```python
from build123d import *

# Parameters (mm, degrees)
SKETCH_1_W               = 20
SKETCH_1_H               = 149.015
SKETCH_1_R               = 2.15
EXTRUDE_1_DEPTH          = 10
SKETCH_2_W               = 20
SKETCH_2_H               = 20
EXTRUDE_2_DEPTH          = 40
SKETCH_3_W               = 20
SKETCH_3_H               = 20
EXTRUDE_3_DEPTH          = 18
CUT_EXTRUDE_1_DEPTH      = 10
CUT_EXTRUDE_1_DEPTH_BACK = 20
SKETCH_5_R               = 2.2
CUT_EXTRUDE_2_DEPTH      = 2
CUT_EXTRUDE_START        = -2
SKETCH_6_R               = 5
SKETCH_6_R_2             = 4.75
CUT_EXTRUDE_3_DEPTH      = 20
SKETCH_7_W               = 20
SKETCH_7_H               = 10
EXTRUDE_4_DEPTH          = 40
CUT_EXTRUDE_5_REACH      = 109.242


with BuildPart() as part:
    # 草图1 → 凸台-拉伸1 (new body)
    with BuildSketch(Plane.XY):
        with Locations((20.013762606, -57.295888527)):
            Rectangle(SKETCH_1_W, SKETCH_1_H)
        with Locations((20, -124.653388527)):
            Circle(SKETCH_1_R, mode=Mode.SUBTRACT)
    extrude(amount=EXTRUDE_1_DEPTH)

    # 草图2 → 凸台-拉伸2 (add)
    with BuildSketch(Plane.XY.offset(10)):
        with Locations((20.013762606, 7.211611473)):
            Rectangle(SKETCH_2_W, SKETCH_2_H)
    extrude(amount=EXTRUDE_2_DEPTH)

    # 草图3 → 凸台-拉伸3 (add)
    with BuildSketch(Plane(origin=(0, 0, 0), x_dir=(-1, 0, 0), z_dir=(0, 0, -1))):
        with Locations((-20.013762606, 7.211611473)):
            Rectangle(SKETCH_3_W, SKETCH_3_H)
    extrude(amount=EXTRUDE_3_DEPTH)

    # 草图4 → 切除-拉伸1 (cut, two sides: drawn at the far end of the back side and taken through both)
    with BuildSketch(Plane.XZ.offset(2.788388527).offset(-CUT_EXTRUDE_1_DEPTH_BACK)):
        Polygon((17.893762606, 50), (30.013762606, 50), (30.013762606, 10), align=None)
        Polygon((17.893762606, -18), (30.013762606, -18), (30.013762606, 0), align=None)
    extrude(amount=CUT_EXTRUDE_1_DEPTH + CUT_EXTRUDE_1_DEPTH_BACK, mode=Mode.SUBTRACT)

    # 草图5 → 切除-拉伸2 (cut)
    with BuildSketch(Plane.ZY.offset(-10.013762606)):
        with Locations(Location((14.7, 7.211611473, 0), (0, 0, 270))):
            Circle(SKETCH_5_R)
        with Locations(Location((40.7, 7.211611473, 0), (0, 0, 270))):
            Circle(SKETCH_5_R)
        with Locations(Location((-11.3, 7.211611473, 0), (0, 0, 270))):
            Circle(SKETCH_5_R)
    extrude(amount=-CUT_EXTRUDE_2_DEPTH, mode=Mode.SUBTRACT)

    # 草图6 → 切除-拉伸3 (cut)
    with BuildSketch(Plane.ZY.offset(-10.013762606).offset(CUT_EXTRUDE_START)):
        with Locations(Location((40.7, 7.211611473, 0), (0, 0, 270))):
            Circle(SKETCH_6_R)
        with Locations(Location((-11.3, 7.211611473, 0), (0, 0, 270))):
            Circle(SKETCH_6_R)
        with Locations(Location((14.7, 7.211611473, 0), (0, 0, 270))):
            Circle(SKETCH_6_R_2)
    extrude(amount=-CUT_EXTRUDE_3_DEPTH, mode=Mode.SUBTRACT)

    # 草图7 → 凸台-拉伸4 (add)
    with BuildSketch(Plane(origin=(0, 0, 0), x_dir=(-1, 0, 0), z_dir=(0, 0, -1))):
        with Locations((-20.013762606, -46.803388527)):
            Rectangle(SKETCH_7_W, SKETCH_7_H)
    extrude(amount=EXTRUDE_4_DEPTH)

    # 草图8 → 切除-拉伸5 (cut, up to next)
    with BuildSketch(Plane(origin=(0, -41.803388527, 0), x_dir=(1, 0, 0), z_dir=(0, 1, 0)), mode=Mode.PRIVATE) as cut_extrude_5_sk1:
        with BuildLine():
            Line((30.013762606, 20), (30.013762606, 40))
            Line((30.013762606, 40), (11.013762606, 40))
            ThreePointArc((11.013762606, 40), (19.239482102, 28.789433521), (30.013762606, 20))
        make_face()
    cut_extrude_5_tool1 = extrude(cut_extrude_5_sk1.sketch, amount=-CUT_EXTRUDE_5_REACH, mode=Mode.PRIVATE) & part.part
    add(cut_extrude_5_tool1.solids().sort_by_distance((23.14433, -41.803389, -32.776655))[0], mode=Mode.SUBTRACT)


solid = part.part
```
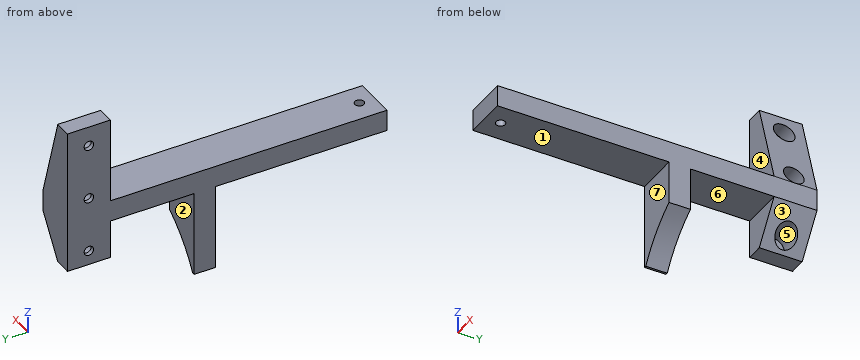
Could you check a few things on this model? Use its own coordinates, in mm. Face numbers are marked on the shaded views. A direction names the side the tool comes from. Round coordinates to 2 decimals unless told otherwise and drop trailing zeros. Order: outer loops, then holes, each group sorted by start corner. A loop starts at its lowest first (then second) coordinate and runs counter-clockwise, first axis right, second up. Notation, with made-up numbers: M 6.25,46 L 46.25,46 A16 cw 46.25,74 Z; hole C 84,18 d7. An arc over 180 degrees is marked long. One line per question, with ' | ' between items. Start each with the question number.
(1) Please list where these lines run through material, in increasing order: line 1 along Y through (x, z) = (17.5, -11.3); line 2 along Y through (x, z) = (21.5, -3); line 3 along Y through (x, z) = (16.5, 14.7).
(2) Thinking about a two-plate mould opening in Z: for the marked faces 5, 6 and 7, which applies, +Z half, -Z half, draft (parallel to the pull), parting line (faces both ways), or undercut?
(3) Suppose I cut it at C-C on z = -11.3. List the corners of the cut face in (x, y) for me.
(4) Suppose I cut it at A-A on z = 40.7. List the corners of the cut face in (x, y) for me.
(5) Suppose I cut it at D-D on x = 16.25. List the corners of the cut face in (y, z) for me, then the cut area to 3 significant figures.
(6) For P1, Ø6, axis at x = 18.5, z = -20.5, coming from the -Y side; P2, Ø11, axis at y = 8.5, z = -12.5, coming from the +X side; P3, Ø1.5, axis at x = 21.5, y = -87, coming from the -Z side, each with a flat end and sliding along its axis, tell me the tip position at first contact or that it passes through.
(7) Suppose I cut it at B-B on y = -44.5. List the corners of the cut face in (x, z) for me, then the cut area to 3 significant figures.
(8) For the marked faces 1, 2, 3 and 4, which set-ups out of +Z, -Z, +X, -X, +Y, -Y let a thin tool reach every point of the face, with its end or its side?
Geometry results:
1) line 1: -51.8 to -41.8, -2.79 to 2.21, 12.21 to 17.21 | line 2: -51.8 to -41.8, -2.79 to 17.21 | line 3: -2.79 to 2.46, 11.96 to 17.21
2) face 5: undercut | face 6: -Z half | face 7: draft
3) outline: M 10.01,-51.8 L 30.01,-51.8 L 30.01,-41.8 L 10.01,-41.8 Z; M 10.01,-2.79 L 22.41,-2.79 L 22.41,2.21 L 12.01,2.21 L 12.01,5.01 L 10.01,5.01 Z; M 10.01,9.41 L 12.01,9.41 L 12.01,12.21 L 22.41,12.21 L 22.41,17.21 L 10.01,17.21 Z
4) outline: M 10.01,-2.79 L 20.71,-2.79 L 20.71,2.21 L 12.01,2.21 L 12.01,5.01 L 10.01,5.01 Z; M 10.01,9.41 L 12.01,9.41 L 12.01,12.21 L 20.71,12.21 L 20.71,17.21 L 10.01,17.21 Z
5) outline: M -131.8,0 L -51.8,0 L -51.8,-32.21 L -41.8,-32.21 L -41.8,0 L -2.79,0 L -2.79,-18 L 17.21,-18 L 17.21,50 L -2.79,50 L -2.79,10 L -131.8,10 Z; hole C 7.21,-11.3 d10; hole C 7.21,40.7 d10; hole C 7.21,14.7 d9.5 | area: 2,740 mm²
6) P1: y = -51.8 | P2: x = 25.13 | P3: z = 0
7) outline: M 10.01,-40 L 11.01,-40 A55 cw 30.01,-20 L 30.01,10 L 10.01,10 Z | area: 778 mm²
8) face 1: -Z, +X, -X, -Y | face 2: -Z, +X, -X | face 3: -Z, +X, +Y | face 4: +Z, +X, -X, -Y
